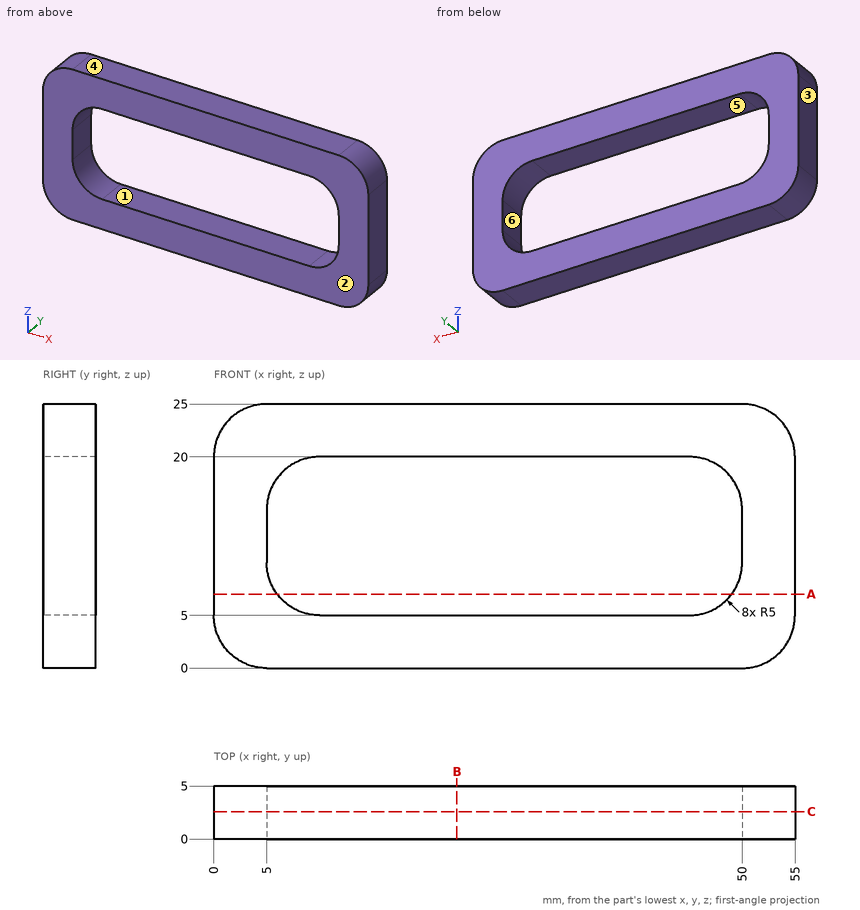
Design review of the part shown in the three views and the two pictorial views. Dimensions are in mm from the part's minimum x, y and z. A direction names the side the tool comes from. Round coordinates to 2 decimals unless told otherwise and drop trailing zeros. Order: outer loops, then holes, each group sorted by start corner. A loop starts at its lowest first (then second) coordinate and runs counter-clockwise, first axis right, second up. Notation, with made-up numbers: (55.25, 45) - (81.25, 45) arc R33 ccw to (81.25, 82) - close; hole circle Ø7 at (-14.75, 18). An arc over 180 degrees is marked (long way). One line per question, with ' | ' between items.
Item 1: Draft analysis for pull direction X (two halves, no side actions). For the marked faces 3, 4, 5 and 6, state which applies: +X half, -X half, draft (parallel to the pull), parting line (faces both ways), or undercut.
Checks:
face 3: -X half | face 4: draft | face 5: undercut | face 6: undercut
Item 2: Machinability: for the marked faces 1 and 2, which of the approach directions +Z, -Z, +X, -X, +Y, -Y give a long, thin tool a straight path to every point of the face, cutting with its end or side? Answer none if there is none.
Checks:
face 1: +Y, -Y | face 2: +Z, -Z, +X, -X, -Y
Item 3: Take a section at C-C, the plane y = 2.6. Write out the cut boundary in (x, z).
Checks:
outline: (0, 5) arc R5 ccw to (5, 0) - (50, 0) arc R5 ccw to (55, 5) - (55, 20) arc R5 ccw to (50, 25) - (5, 25) arc R5 ccw to (0, 20) - close; hole (5, 10) arc R5 ccw to (10, 5) - (45, 5) arc R5 ccw to (50, 10) - (50, 15) arc R5 ccw to (45, 20) - (10, 20) arc R5 ccw to (5, 15) - close
Item 4: Take a section at A-A, the plane z = 7. Write out the cut boundary in (x, y).
Checks:
outline: (0, 0) - (6, 0) - (6, 5) - (0, 5) - close; (49, 0) - (55, 0) - (55, 5) - (49, 5) - close
Item 5: Wall thickness on line 1 (Z direction, x = 24, y = 4.3); line 2 (X direction, y = 2.95, z = 13.75); line 3 (X direction, y = 3.55, z = 17.25): over which ranges is each line inside the solid? List them lowest first. Write a range as [from, to].
Checks:
line 1: [0, 5], [20, 25] | line 2: [0, 5], [50, 55] | line 3: [0, 5.53], [49.47, 55]
Item 6: Take a section at B-B, the plane x = 23. Write out the cut boundary in (y, z), then the cut area to 3 significant figures.
Checks:
outline: (0, 0) - (5, 0) - (5, 5) - (0, 5) - close; (0, 20) - (5, 20) - (5, 25) - (0, 25) - close | area: 50.0 mm²
